Could you check a few things on this drawing? It's one solid part, dimensions in mm from its lowest x, y, z. Round coordinates to 2 decimals unless told otherwise and drop trailing zeros. Loops run counter-clockwise (first coordinate to the right, second up) from the corner with the lowest first, then second, coordinate; pieces in that order, holes last. Notation, with made-up numbers: M -33,-13.75 L -7,-13.75 A12 cw -7,8.25 Z; hole C -26.75,-21 d4. An arc over 180 degrees is marked long. Put each result on its own line as item: value. Start each with the question number.
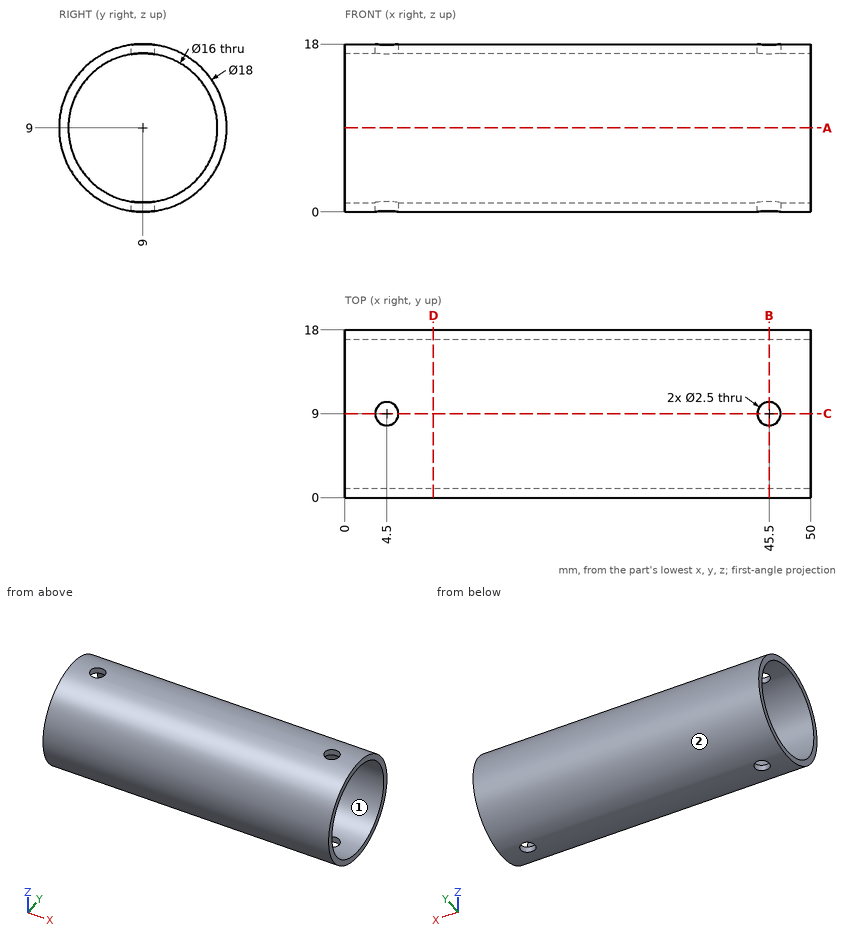
1) If we mould it in two halves opening along Y, with no side actions, what happens to the marked faces 1 and 2? For each: pulls with the +Y half, pulls with the -Y half, needs draft (parallel to the pull), parting line crosses it, or undercut.
2) I'm going to push flat-ended pins straight in: P1, Ø4, axis at x = 18.5, y = 15.5, coming from the +Z side; P2, Ø1, axis at x = 37, y = 2, coming from the -Z side; P3, Ø1, axis at x = 20.5, z = 6, coming from the -Y side. Where does each tip first touch, or does it pass through?
3) If I drill on probe 1 along Y at (x, z) = (37, 15.5); probe 2 along Y at (x, z) = (4, 13.75); probe 3 along Z at (x, y) = (32, 12.75), over which ranges is the centre line in solid material (lowest first)? Write a range as from..to.
4) Suppose I cut it at B-B (x = 45.5). Write out the boundary of the cut face in (y, z).
5) Suppose I cut it at A-A (z = 9). Write out the boundary of the cut face in (x, y).
6) Suppose I cut it at C-C (y = 9). Write out the boundary of the cut face in (x, z).
7) Suppose I cut it at D-D (x = 9.5). Write out the boundary of the cut face in (y, z), plus the area to 3 significant figures.
Results are:
1. face 1: undercut
1. face 2: parting line crosses it
2. P1: z = 16.79
2. P2: z = 2.78
2. P3: y = 0.35
3. probe 1: 2.78..4.34, 13.66..15.22
3. probe 2: 1.36..2.56, 15.44..16.64
3. probe 3: 0.82..1.93, 16.07..17.18
4. outline: M 7.75,0.09 L 7.75,1.1 A8 cw 7.75,16.9 L 7.75,17.91 A9 ccw Z; M 10.25,0.09 A9 ccw 10.25,17.91 L 10.25,16.9 A8 cw 10.25,1.1 Z
5. outline: M 0,0 L 50,0 L 50,1 L 0,1 Z; M 0,17 L 50,17 L 50,18 L 0,18 Z
6. outline: M 0,0 L 3.25,0 L 3.25,1 L 0,1 Z; M 0,17 L 3.25,17 L 3.25,18 L 0,18 Z; M 5.75,0 L 44.25,0 L 44.25,1 L 5.75,1 Z; M 5.75,17 L 44.25,17 L 44.25,18 L 5.75,18 Z; M 46.75,0 L 50,0 L 50,1 L 46.75,1 Z; M 46.75,17 L 50,17 L 50,18 L 46.75,18 Z
7. outline: C 9,9 d18; hole C 9,9 d16
7. area: 53.4 mm²
